For this review, take the finished solid that the model builds, in its own axes (mm). Coordinates: 2 decimals unless noted, no trailing zeros. Write each loop counter-clockwise with the first axis right and the second up, starting at its lowest first coordinate (ties: lowest second). Pieces come first, ordered by that corner, then holes. Notation, with made-up numbers: (55, -38.75) - (88, -38.75) arc R22 cw to (88, -7.75) - close; hole circle Ø9 at (21, 6). An arc over 180 degrees is marked (long way). Use one line per item in the form item = value. Start each with the question number.
1) Mouldability with a two-part tool opening along Z and no side actions: class faces 1 (the cylindrical face through (7.436, -0.976, 19.72)), 2 (the flat face through (0, 10, 0)), 3 (the cylindrical face through (-12.435, 13.439, 21.201)) as pulls with the +Z half, pulls with the -Z half, needs draft (parallel to the pull), parting line crosses it, or undercut.
2) We need section B-B (x = 0). Give the boundary of the cut face in (y, z), plus the area to 3 significant figures.
3) Insertion check: P1, Ø5, axis at y = 0, z = 25, coming from the +X side; P2, Ø4, axis at x = -16, y = 16, coming from the -Z side; P3, Ø1.5, axis at y = 4, z = 20, coming from the -X side. Each pin has a flat end and moves straight along its axis. Give the tip position at first contact, or say it passes through.
4) We need section C-C (z = 33). Give the boundary of the cut face in (x, y).
5) We need section D-D (y = 16). Give the boundary of the cut face in (x, z).
6) For L1, parallel to X at y = 17.25, z = 20; L2, parallel to Z at x = -16.25, y = 13.75; L3, parallel to X at y = 22, z = 19, list the stretches that pass through material, from the lowest coordinate up. Write a range as from..to.
7) We need section A-A (z = 20). Give the boundary of the cut face in (x, y), plus the area to 3 significant figures.
```python
from build123d import *

# Parameters (mm, degrees)
F1_DEPTH    = 40
F2_T1_DEPTH = 40
F3_R        = 4
F4_DEPTH    = 30


# Not quite as in the source:
# - a fillet or chamfer that OpenCascade refuses, or shapes differently, is made with other operations: its cross-section is extruded or revolved along the edge and cut away or added


with BuildPart() as f1:
    # F0 (on Top) → F1 (new body)
    with BuildSketch(Plane.XY):
        with BuildLine():
            Line((10, 7.5), (0, 7.5))
            Line((0, 7.5), (-10, 7.5))
            ThreePointArc((-10, 7.5), (-3.9528470752, -11.8585412256), (12.5, 0))
            ThreePointArc((12.5, 0), (11.8585412256, 3.9528470752), (10, 7.5))
        make_face()
        with BuildLine():
            ThreePointArc((0, 7.5), (5.3033008589, 5.3033008589), (7.5, 0))
            ThreePointArc((7.5, 0), (-5.3033008589, -5.3033008589), (0, 7.5))
        make_face(mode=Mode.SUBTRACT)
        with BuildLine():
            Line((0, 12.5), (0, 7.5))
            Line((0, 7.5), (10, 7.5))
            ThreePointArc((10, 7.5), (5.5901699437, 11.1803398875), (0, 12.5))
        make_face()
        with BuildLine():
            ThreePointArc((0, 12.5), (5.5901699437, 11.1803398875), (10, 7.5))
            Line((10, 7.5), (25, 7.5))
            Line((25, 7.5), (25, 24))
            Line((25, 24), (0, 24))
            Line((0, 24), (0, 12.5))
        make_face()
        with BuildLine():
            ThreePointArc((-10, 7.5), (-5.5901699437, 11.1803398875), (0, 12.5))
            Line((0, 12.5), (0, 24))
            Line((0, 24), (-25, 24))
            Line((-25, 24), (-25, 7.5))
            Line((-25, 7.5), (-10, 7.5))
        make_face()
        with BuildLine():
            Line((-10, 7.5), (0, 7.5))
            Line((0, 7.5), (0, 12.5))
            ThreePointArc((0, 12.5), (-5.5901699437, 11.1803398875), (-10, 7.5))
        make_face()
    extrude(amount=F1_DEPTH)

    # F2: fillet of radius 15 on 2 edges, made by hand

    # F2_s2 → F2_t1 (join)
    with BuildSketch(Plane.XY):
        with BuildLine():
            ThreePointArc((12.0354995182, -3.375907485), (16.8376373335, 4.064804959), (25, 7.5))
            Line((25, 7.5), (10, 7.5))
            ThreePointArc((10, 7.5), (12.2866655631, 2.2995324178), (12.0354995182, -3.375907485))
        make_face()
        with BuildLine():
            ThreePointArc((-25, 7.5), (-16.8376373335, 4.064804959), (-12.0354995182, -3.375907485))
            ThreePointArc((-12.0354995182, -3.375907485), (-12.2866655631, 2.2995324178), (-10, 7.5))
            Line((-10, 7.5), (-25, 7.5))
        make_face()
    extrude(amount=F2_T1_DEPTH)

    # F3 (on Front) → F4 (cut, symmetric)
    with BuildSketch(Plane.XZ):
        with Locations((16.25, 20)):
            Circle(F3_R)
        with Locations((-16.25, 20)):
            Circle(F3_R)
    extrude(amount=F4_DEPTH, both=True, mode=Mode.SUBTRACT)


solid = f1.part
```
Determined:
q1.face_1 = needs draft
q1.face_2 = pulls with the -Z half
q1.face_3 = undercut
q2.outline = (-12.5, 0) - (-7.5, 0) - (-7.5, 40) - (-12.5, 40) - close; (7.5, 0) - (24, 0) - (24, 40) - (7.5, 40) - close
q2.area = 860 mm²
q3.P1 = 15.23
q3.P2 = 0
q3.P3 = -12.32
q4.outline = (-25, 7.5) arc R15 cw to (-12.04, -3.38) arc R12.5 ccw to (12.04, -3.38) arc R15 cw to (25, 7.5) - (25, 24) - (-25, 24) - close; hole circle Ø15 at (0, 0)
q5.outline = (-25, 0) - (25, 0) - (25, 40) - (-25, 40) - close; hole circle Ø8 at (-16.25, 20); hole circle Ø8 at (16.25, 20)
q6.L1 = -25..-20.25, -12.25..12.25, 20.25..25
q6.L2 = 0..16, 24..40
q6.L3 = -25..-20.12, -12.38..12.38, 20.12..25
q7.outline = (-25, 7.5) arc R15 cw to (-20.25, 6.22) - (-20.25, 24) - (-25, 24) - close; (-12.25, -2.68) arc R15 cw to (-12.04, -3.38) arc R12.5 ccw to (12.04, -3.38) arc R15 cw to (12.25, -2.68) - (12.25, 24) - (-12.25, 24) - close; (20.25, 6.22) arc R15 cw to (25, 7.5) - (25, 24) - (20.25, 24) - close; hole circle Ø15 at (0, 0)
q7.area = 817 mm²
